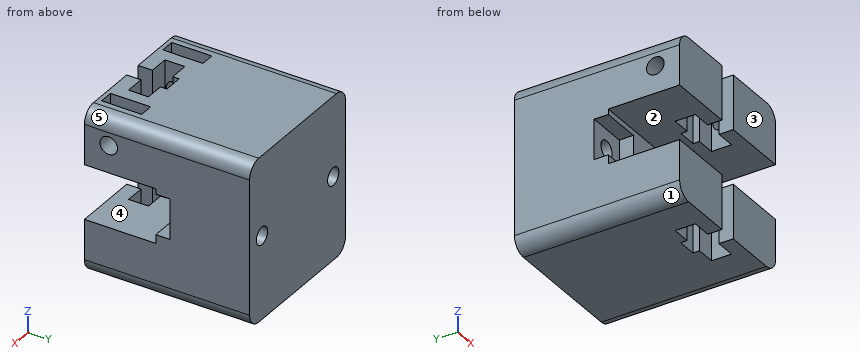
from build123d import *

# Parameters (mm, degrees)
F1_DEPTH  = 29
F2_W      = 26.8
F2_H      = 9.666666
F3_DEPTH  = 12.7
F4_R      = 2.54
F5_R      = 1.5625
F6_DEPTH  = 16.689
F7_W      = 7.14375
F7_H      = 7.14375
F8_DEPTH  = 2.5
F11_R     = 1.5625
F12_DEPTH = 26.801
F15_W     = 2.5
F15_H     = 7.14375
F16_DEPTH = 7.82


with BuildPart() as f1:
    # F0 (on Top) → F1 (new body)
    with BuildSketch(Plane.XY):
        Polygon((-11.8125, 0), (0, 0), (0, 29.389), (-26.8, 29.389), (-26.8, 0), (-14.9875, 0), (-14.9875, 2.54), (-18.48, 2.54), (-18.48, 6.096), (-15.1145, 6.096), (-15.1145, 7.239), (-11.6855, 7.239), (-11.6855, 6.096), (-8.32, 6.096), (-8.32, 2.54), (-11.8125, 2.54), align=None)
    extrude(amount=F1_DEPTH)

    # F2 (on face) → F3 (cut)
    with BuildSketch(Plane.XZ):
        with Locations((-13.4, 14.5)):
            Rectangle(F2_W, F2_H)
    extrude(amount=-F3_DEPTH, mode=Mode.SUBTRACT)

    # F4
    f4_edges = [f1.edges().sort_by_distance(p)[0] for p in [
        (0, 14.6945, 29),
        (-26.8, 14.6945, 29),
        (-26.8, 14.6945, 0),
        (0, 14.6945, 0),
    ]]
    fillet(f4_edges, radius=F4_R)

    # F5 (on face) → F6 (cut, through all)
    with BuildSketch(Plane(origin=(0, 29.389, 0), x_dir=(-1, 0, 0), z_dir=(0, 1, 0))):
        with Locations((3.45, 14.8)):
            Circle(F5_R)
        with Locations((23.35, 14.8)):
            Circle(F5_R)
    extrude(amount=-F6_DEPTH, mode=Mode.SUBTRACT)

    # F7 (on face) → F8 (cut)
    with BuildSketch(Plane.XZ.offset(-12.7)):
        with Locations((-23.35, 14.8)):
            Rectangle(F7_W, F7_H)
        with Locations((-3.45, 14.8)):
            Rectangle(F7_W, F7_H)
    extrude(amount=-F8_DEPTH, mode=Mode.SUBTRACT)

    # F11 (on face) → F12 (cut, through all)
    with BuildSketch(Plane.YZ):
        with Locations((4.318, 24.158125)):
            Circle(F11_R)
    extrude(amount=-F12_DEPTH, mode=Mode.SUBTRACT)

    # F15 (on face) → F16 (cut)
    with BuildSketch(Plane.XY.offset(29)):
        with Locations((-4.8475, 4.318)):
            Rectangle(F15_W, F15_H)
        with Locations((-21.9525, 4.318)):
            Rectangle(F15_W, F15_H)
    extrude(amount=-F16_DEPTH, mode=Mode.SUBTRACT)


solid = f1.part
Verification items for the finished model (mm, model axes). Face numbers are marked on the shaded views. A direction names the side the tool comes from. Coordinates: 2 decimals unless noted, no trailing zeros. Order: outer loops, then holes, each group sorted by start corner. A loop starts at its lowest first (then second) coordinate and runs counter-clockwise, first axis right, second up.
Item 1: Release check for a two-part mould opening along Z. For the marked faces 1, 2 and 3 record: +Z half, -Z half, draft (parallel to the pull), parting line (faces both ways), or undercut.
Filled in:
face 1: -Z half
face 2: undercut
face 3: draft
Item 2: Section check C-C, the plane z = 14.8. Enter the section's corners in (x, y), then the cut area to 3 significant figures.
Filled in:
outline: (-26.8, 15.2) - (-24.91, 15.2) - (-24.91, 29.39) - (-26.8, 29.39) - close; (-21.79, 15.2) - (-19.78, 15.2) - (-19.78, 12.7) - (-7.02, 12.7) - (-7.02, 15.2) - (-5.01, 15.2) - (-5.01, 29.39) - (-21.79, 29.39) - close; (-1.89, 15.2) - (0, 15.2) - (0, 29.39) - (-1.89, 29.39) - close
area: 323 mm2
Item 3: Access from +Z, -Z, +X, -X, +Y, -Y to the whole of each face (thin tool, end or side, straight path). Record for the marked faces 4 and 5.
Filled in:
face 4: +X, -X, -Y
face 5: +Z, +X, +Y, -Y
Item 4: Section check D-D, the plane y = 11. Enter the section's corners in (x, z), then the cut area to 3 significant figures.
Filled in:
outline: (-26.8, 2.54) arc R2.54 ccw to (-24.26, 0) - (-2.54, 0) arc R2.54 ccw to (0, 2.54) - (0, 9.67) - (-26.8, 9.67) - close; (-26.8, 19.33) - (0, 19.33) - (0, 26.46) arc R2.54 ccw to (-2.54, 29) - (-24.26, 29) arc R2.54 ccw to (-26.8, 26.46) - close
area: 513 mm2
Item 5: Depth check by flat-ended pin: pin 1 (0.8 mm diameter, centred on y = 14.5, z = 14.5, fed in from -X); pin 2 (7.5 mm diameter, centred on x = -3.5, z = 15.5, fed in from -Y); pin 3 (1.2 mm diameter, centred on x = -4.5, y = 3.5, fed in from +Z). Enter the tip coordinate at first touch or a pass-through.
Filled in:
pin 1: stops at x = -19.78
pin 2: stops at y = 12.7
pin 3: stops at z = 21.18
Item 6: Section check A-A, the plane x = -17.25. Enter the section's corners in (y, z).
Filled in:
outline: (0, 0) - (2.54, 0) - (2.54, 9.67) - (0, 9.67) - close; (0, 19.33) - (2.54, 19.33) - (2.54, 29) - (0, 29) - close; (6.1, 0) - (29.39, 0) - (29.39, 29) - (6.1, 29) - (6.1, 19.33) - (12.7, 19.33) - (12.7, 9.67) - (6.1, 9.67) - close
Item 7: Section check B-B, the plane y = 27.75. Give the number of separate pieces and of enclosed holes in the cut face, then the cut area to 3 significant figures.
Filled in:
separate pieces: 1
enclosed holes: 2
area: 756 mm2
Item 8: Material ranges on L1, parallel to Z at x = -23.35, y = 19; L2, parallel to Y at x = -16.25, z = 27.25; L3, parallel to X at y = 4.5, z = 22.5, recorded low to high.
Filled in:
L1: z = 0 to 13.24, 16.36 to 29
L2: y = 0 to 2.54, 6.1 to 29.39
L3: x = -26.8 to -23.2, -20.7 to -18.48, -8.32 to -6.1, -3.6 to 0
